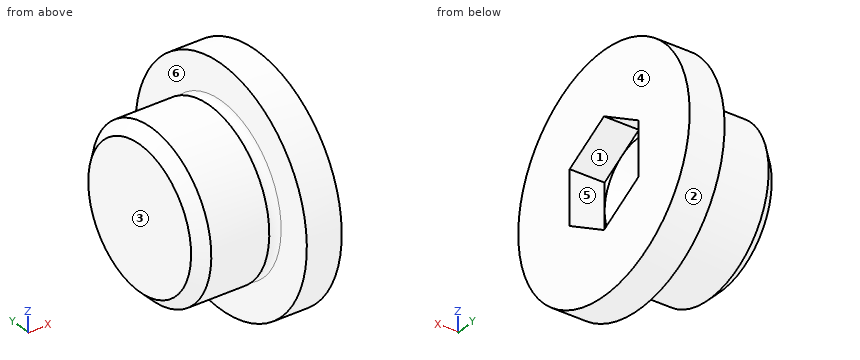
from build123d import *

# Parameters (mm, degrees)
ENL_V_MAT_EXTRU_1_DEPTH = 3
CHANFREIN1_SIZE         = 1


with BuildPart() as part:
    # Esquisse1 → Révolution1 (revolve)
    with BuildSketch(Plane.XY, mode=Mode.PRIVATE) as r_volution1_sk:
        with BuildLine():
            Line((0, 0), (0, 7))
            Line((0, 7), (5.983785808, 7))
            ThreePointArc((5.983785808, 7), (6.491892904, 6.491892904), (7, 7))
            Line((7, 7), (7, 10))
            Line((7, 10), (10, 10))
            Line((10, 10), (10, 0))
            Line((10, 0), (0, 0))
        make_face()
    revolve(r_volution1_sk.sketch.rotate(Axis((0, 0, 0), (1, 0, 0)), 90), axis=Axis((0, 0, 0), (1, 0, 0)))

    # Esquisse5 → Diamètre du perçage Ø8.0 (8)1 (revolve, cut)
    with BuildSketch(Plane(origin=(10, 0, 0), x_dir=(0, 0, -1), z_dir=(0, 1, 0))):
        Polygon((0, 0), (0, 5.403442476), (4, 3), (4, 0), align=None)
    revolve(axis=Axis((16.35, 0, 0), (-1, 0, 0)), mode=Mode.SUBTRACT)

    # Esquisse3 → Enlèv. mat.-Extru.1 (cut)
    with BuildSketch(Plane(origin=(10, 0, 0), x_dir=(0, 0, -1), z_dir=(1, 0, 0))):
        Polygon((-4.618802154, 0), (-2.309401077, 4), (2.309401077, 4), (4.618802154, 0), (2.309401077, -4), (-2.309401077, -4), align=None)
    extrude(amount=-ENL_V_MAT_EXTRU_1_DEPTH, mode=Mode.SUBTRACT)

    # Chanfrein1
    chanfrein1_edges = [part.edges().sort_by_distance(p)[0] for p in [
        (0, 0, -7),
    ]]
    chamfer(chanfrein1_edges, length=CHANFREIN1_SIZE)


solid = part.part
Could you check a few things on this model? Use its own coordinates, in mm. Face numbers are marked on the shaded views. A direction names the side the tool comes from. Coordinates: 2 decimals unless noted, no trailing zeros. Order: outer loops, then holes, each group sorted by start corner. A loop starts at its lowest first (then second) coordinate and runs counter-clockwise, first axis right, second up.
Q1. Suppose I cut it at B-B on x = 0.5. Please give me the cut outline in (y, z), and give its area (3 significant figures).
Q2. Will these pins go through, and if not, where does the flat tip stop? pin 1 (3 mm diameter, centred on x = 4, y = -3.5, fed in from -Z); pin 2 (1.5 mm diameter, centred on x = 8.5, y = -4.5, fed in from -Z); pin 3 (4 mm diameter, centred on x = 4, z = -6, fed in from -Y).
Q3. Please list where these lines run through material, in increasing order: L1, parallel to X at y = 4.75, z = 8; L2, parallel to Y at x = 8.5, z = 1.25; L3, parallel to Y at x = 9, z = 4.5.
Q4. Suppose I cut it at A-A on x = 7.25. Please give me the cut outline in (y, z), and give its area (3 significant figures).
Q5. Which directions (+Z, -Z, +X, -X, +Y, -Y) give clear straight access to the entire face, cutting with the end or side of a thin tool? Please do the marked faces 4, 5 and 6.
Q6. Thinking about a two-plate mould opening in Y: for the marked faces 1, 2 and 3, which applies, released by +Y, released by -Y, zero draft, split by the parting line, or undercut?
Q7. Suppose I cut it at C-C on y = 8.25. Please give me the cut outline in (x, z).
Q8. Suppose I cut it at D-D on x = 5. Please give me the cut outline in (y, z), and give its area (3 significant figures).
Answer:
1. outline: circle Ø13 at (0, 0)
1. area: 133 mm2
2. pin 1: stops at z = -6.71
2. pin 2: stops at z = -9.27
2. pin 3: stops at y = -5.74
3. L1: x = 7 to 10
3. L2: y = -9.92 to -4, 4 to 9.92
3. L3: y = -8.93 to -0.21, 0.21 to 8.93
4. outline: circle Ø20 at (0, 0); hole (-4, -2.31) - (0, -4.62) - (4, -2.31) - (4, 2.31) - (0, 4.62) - (-4, 2.31) - close
4. area: 259 mm2
5. face 4: +Z, -Z, +X, +Y, -Y
5. face 5: +X
5. face 6: -X
6. face 1: undercut
6. face 2: split by the parting line
6. face 3: zero draft
7. outline: (7, -5.65) - (10, -5.65) - (10, 5.65) - (7, 5.65) - close
8. outline: circle Ø14 at (0, 0); hole circle Ø1.34 at (0, 0)
8. area: 153 mm2
